Verification items for the finished model (mm, model axes). Face numbers are marked on the shaded views. A direction names the side the tool comes from. Round coordinates to 2 decimals unless told otherwise and drop trailing zeros. Order: outer loops, then holes, each group sorted by start corner. A loop starts at its lowest first (then second) coordinate and runs counter-clockwise, first axis right, second up.
```python
from build123d import *

# Parameters (mm, degrees)
SKETCH1_W             = 80
SKETCH1_H             = 40
SKETCH1_R             = 1.55
BOSS_EXTRUDE1_DEPTH   = 5
SKETCH1_W_2           = 40
SKETCH1_H_2           = 80
BOSS_EXTRUDE1_2_DEPTH = 5
BOSS_EXTRUDE1_3_DEPTH = 5
BOSS_EXTRUDE1_4_DEPTH = 5
SKETCH1_4_W           = 40
SKETCH1_4_H           = 40
BOSS_EXTRUDE2_DEPTH   = 310
CHAMFER1_SIZE         = 50
CHAMFER2_SIZE         = 50
BOSS_EXTRUDE3_START   = 180
SKETCH2_R             = 1.55
BOSS_EXTRUDE3_DEPTH   = 7.5
CHAMFER7_SIZE         = 10
SKETCH3_W             = 15
SKETCH3_H             = 15
BOSS_EXTRUDE4_DEPTH   = 20
SKETCH4_W             = 40
SKETCH4_H             = 22.28
BOSS_EXTRUDE5_DEPTH   = 5
CHAMFER8_SIZE         = 22
CHAMFER8_SIZE2        = 29.194986076


# Some blends are built 0.0001 mm under size
with BuildPart() as part:
    # Sketch1 → Boss-Extrude1 (new body)
    with BuildSketch(Plane(origin=(0, 0, 0), x_dir=(1, 0, 0), z_dir=(0, 1, 0))):
        with Locations((40, 20)):
            Rectangle(SKETCH1_W, SKETCH1_H)
        with Locations(Location((74, 6, 0), (0, 0, 270))):
            Circle(SKETCH1_R, mode=Mode.SUBTRACT)
        with Locations(Location((74, 34, 0), (0, 0, 270))):
            Circle(SKETCH1_R, mode=Mode.SUBTRACT)
    extrude(amount=BOSS_EXTRUDE1_DEPTH)



with BuildPart() as body_2:
    # Sketch1 → Boss-Extrude1 2 (new body)
    with BuildSketch(Plane(origin=(0, 0, 0), x_dir=(1, 0, 0), z_dir=(0, 1, 0))):
        with Locations((-20, 80)):
            Rectangle(SKETCH1_W_2, SKETCH1_H_2)
        with Locations(Location((-34, 114, 0), (0, 0, 270))):
            Circle(SKETCH1_R, mode=Mode.SUBTRACT)
        with Locations(Location((-6, 114, 0), (0, 0, 270))):
            Circle(SKETCH1_R, mode=Mode.SUBTRACT)
    extrude(amount=BOSS_EXTRUDE1_2_DEPTH)


with BuildPart() as body_3:
    # Sketch1 → Boss-Extrude1 3 (new body)
    with BuildSketch(Plane(origin=(0, 0, 0), x_dir=(1, 0, 0), z_dir=(0, 1, 0))):
        with Locations((-80, 20)):
            Rectangle(SKETCH1_W, SKETCH1_H)
        with Locations(Location((-114, 6, 0), (0, 0, 270))):
            Circle(SKETCH1_R, mode=Mode.SUBTRACT)
        with Locations(Location((-114, 34, 0), (0, 0, 270))):
            Circle(SKETCH1_R, mode=Mode.SUBTRACT)
    extrude(amount=BOSS_EXTRUDE1_3_DEPTH)


with BuildPart() as body_4:
    # Sketch1 → Boss-Extrude1 4 (new body)
    with BuildSketch(Plane(origin=(0, 0, 0), x_dir=(1, 0, 0), z_dir=(0, 1, 0))):
        with Locations((-20, -40)):
            Rectangle(SKETCH1_W_2, SKETCH1_H_2)
        with Locations(Location((-34, -74, 0), (0, 0, 270))):
            Circle(SKETCH1_R, mode=Mode.SUBTRACT)
        with Locations(Location((-6, -74, 0), (0, 0, 270))):
            Circle(SKETCH1_R, mode=Mode.SUBTRACT)
    extrude(amount=BOSS_EXTRUDE1_4_DEPTH)


with BuildPart() as part_1:
    add(part.part)

    add(body_2.part)  # Boss-Extrude2 merges body 2

    add(body_3.part)  # Boss-Extrude2 merges body 3

    add(body_4.part)  # Boss-Extrude2 merges body 4
    # Sketch1<4> → Boss-Extrude2 (add)
    with BuildSketch(Plane(origin=(0, 0, 0), x_dir=(1, 0, 0), z_dir=(0, 1, 0))):
        with Locations((-20, 20)):
            Rectangle(SKETCH1_4_W, SKETCH1_4_H)
    extrude(amount=BOSS_EXTRUDE2_DEPTH)

    # Chamfer1
    # the kernel refuses this chamfer: 50 mm, written as the material it adds along each edge
    with BuildSketch(Plane(origin=(0, 5, -40), x_dir=(1, 0, 0), z_dir=(0, 0, 1)), Plane(origin=(-40, 5, 0), x_dir=(-1, 0, 0), z_dir=(0, 0, -1))) as chamfer1_piece_1:
        Polygon((CHAMFER1_SIZE, 0), (0, CHAMFER1_SIZE), (0, 0), align=None)
    extrude(amount=40)

    # Chamfer2
    chamfer2_edges = [part_1.edges().sort_by_distance(p)[0] for p in [
        (-20, 5, -40),
        (-20, 5, 0),
    ]]
    chamfer(chamfer2_edges, length=CHAMFER2_SIZE - 0.0001)  # a hair under: the kernel refuses the full size

    # Sketch2 → Boss-Extrude3 (add)
    with BuildSketch(Plane(origin=(0, 0, 0), x_dir=(1, 0, 0), z_dir=(0, 1, 0)).offset(BOSS_EXTRUDE3_START)):
        Polygon((-64.25, 76.68), (-44.25, 76.68), (-44.25, 51.75), (-32.5, 40), (-7.5, 40), (4.25, 51.75), (4.25, 76.68), (24.25, 76.68), (24.25, 26.68), (-40, 26.68), (-64.25, 26.68), align=None)
        with Locations(Location((-54.25, 71.68, 0), (0, 0, 270))):
            Circle(SKETCH2_R, mode=Mode.SUBTRACT)
        with Locations(Location((14.25, 71.68, 0), (0, 0, 270))):
            Circle(SKETCH2_R, mode=Mode.SUBTRACT)
        with Locations(Location((-54.25, 31.68, 0), (0, 0, 270))):
            Circle(SKETCH2_R, mode=Mode.SUBTRACT)
        with Locations(Location((14.25, 31.68, 0), (0, 0, 270))):
            Circle(SKETCH2_R, mode=Mode.SUBTRACT)
    extrude(amount=BOSS_EXTRUDE3_DEPTH)

    # Chamfer7
    # the kernel refuses this chamfer: 10 mm, written as the material it adds along each edge
    with BuildSketch(Plane(origin=(-40, 187.5, -26.68), x_dir=(0, 1, 0), z_dir=(0, 0, -1))) as chamfer7_piece_1_section:
        Polygon((CHAMFER7_SIZE, 0), (0, -CHAMFER7_SIZE), (0, 0), align=None)
    chamfer7_piece_1 = extrude(amount=39.03682988, mode=Mode.PRIVATE)
    chamfer7_piece_1 = split(chamfer7_piece_1, bisect_by=Plane(origin=(-29.59, 187.5, -37.09), z_dir=(-0.7071067811865485, 0, 0.7071067811865467)), keep=Keep.TOP, mode=Mode.PRIVATE)
    chamfer7_piece_1 = split(chamfer7_piece_1, bisect_by=Plane(origin=(-40, 199.16, -38.34), z_dir=(0, -0.7071067811865476, 0.7071067811865476)), keep=Keep.TOP, mode=Mode.PRIVATE)
    add(chamfer7_piece_1)
    with BuildSketch(Plane(origin=(0, 187.5, -65.71682988), x_dir=(0, 1, 0), z_dir=(0, 0, 1))) as chamfer7_piece_2_section:
        Polygon((CHAMFER7_SIZE, 0), (0, -CHAMFER7_SIZE), (0, 0), align=None)
    chamfer7_piece_2 = extrude(amount=39.03682988, mode=Mode.PRIVATE)
    chamfer7_piece_2 = split(chamfer7_piece_2, bisect_by=Plane(origin=(9.10841494, 187.5, -56.60841494), z_dir=(0.7071067811865488, 0, 0.7071067811865462)), keep=Keep.TOP, mode=Mode.PRIVATE)
    chamfer7_piece_2 = split(chamfer7_piece_2, bisect_by=Plane(origin=(0, 179.64158506, -57.85841494), z_dir=(0, -0.7071067811865476, 0.7071067811865476)), keep=Keep.TOP, mode=Mode.PRIVATE)
    add(chamfer7_piece_2)
    with BuildSketch(Plane(origin=(-33.21682988, 187.5, -40), x_dir=(0, 1, 0), z_dir=(1, 0, 0))) as chamfer7_piece_3_section:
        Polygon((CHAMFER7_SIZE, 0), (0, -CHAMFER7_SIZE), (0, 0), align=None)
    chamfer7_piece_3 = extrude(amount=58.933659759, mode=Mode.PRIVATE)
    chamfer7_piece_3 = split(chamfer7_piece_3, bisect_by=Plane(origin=(-32.85841494, 187.5, -40.35841494), z_dir=(-0.7071067811865485, 0, 0.7071067811865467)), keep=Keep.TOP, mode=Mode.PRIVATE)
    add(chamfer7_piece_3)
    with BuildSketch(Plane(origin=(-33.21682988, 187.5, -40), x_dir=(0, 1, 0), z_dir=(1, 0, 0))) as chamfer7_piece_4_section:
        Polygon((CHAMFER7_SIZE, 0), (0, -CHAMFER7_SIZE), (0, 0), align=None)
    chamfer7_piece_4 = extrude(amount=58.933659759, mode=Mode.PRIVATE)
    chamfer7_piece_4 = split(chamfer7_piece_4, bisect_by=Plane(origin=(-20.35841494, 187.5, -27.14158506), z_dir=(0.7071067811865488, 0, 0.7071067811865462)), keep=Keep.TOP, mode=Mode.PRIVATE)
    chamfer7_piece_4 = split(chamfer7_piece_4, bisect_by=Plane(origin=(-11.60841494, 209.10841494, -40), z_dir=(-0.7071067811865476, -0.7071067811865476, 0)), keep=Keep.TOP, mode=Mode.PRIVATE)
    add(chamfer7_piece_4)
    with BuildSketch(Plane(origin=(-65.71682988, 187.5, -40), x_dir=(0, 1, 0), z_dir=(1, 0, 0))) as chamfer7_piece_5_section:
        Polygon((CHAMFER7_SIZE, 0), (0, -CHAMFER7_SIZE), (0, 0), align=None)
    chamfer7_piece_5 = extrude(amount=58.933659759, mode=Mode.PRIVATE)
    chamfer7_piece_5 = split(chamfer7_piece_5, bisect_by=Plane(origin=(-49.10841494, 187.5, -56.60841494), z_dir=(-0.7071067811865485, 0, 0.7071067811865467)), keep=Keep.TOP, mode=Mode.PRIVATE)
    chamfer7_piece_5 = split(chamfer7_piece_5, bisect_by=Plane(origin=(-57.85841494, 179.64158506, -40), z_dir=(0.7071067811865476, -0.7071067811865476, 0)), keep=Keep.TOP, mode=Mode.PRIVATE)
    add(chamfer7_piece_5)
    with BuildSketch(Plane(origin=(-65.71682988, 187.5, -40), x_dir=(0, 1, 0), z_dir=(1, 0, 0))) as chamfer7_piece_6_section:
        Polygon((CHAMFER7_SIZE, 0), (0, -CHAMFER7_SIZE), (0, 0), align=None)
    chamfer7_piece_6 = extrude(amount=58.933659759, mode=Mode.PRIVATE)
    chamfer7_piece_6 = split(chamfer7_piece_6, bisect_by=Plane(origin=(-36.60841494, 187.5, -10.89158506), z_dir=(0.7071067811865488, 0, 0.7071067811865462)), keep=Keep.TOP, mode=Mode.PRIVATE)
    add(chamfer7_piece_6)



with BuildPart() as body_2_2:
    # Sketch3 → Boss-Extrude4 (new body)
    with BuildSketch(Plane(origin=(0, 310, 0), x_dir=(1, 0, 0), z_dir=(0, 1, 0))):
        with Locations((-20, 54.78)):
            Rectangle(SKETCH3_W, SKETCH3_H)
    extrude(amount=BOSS_EXTRUDE4_DEPTH)


with BuildPart() as part_2:
    add(part_1.part)

    add(body_2_2.part)  # Boss-Extrude5 merges body 2 2
    # Sketch4 → Boss-Extrude5 (add)
    with BuildSketch(Plane(origin=(0, 310, 0), x_dir=(1, 0, 0), z_dir=(0, 1, 0))):
        with Locations((-20, 51.14)):
            Rectangle(SKETCH4_W, SKETCH4_H)
    extrude(amount=-BOSS_EXTRUDE5_DEPTH)

    # Chamfer8
    chamfer8_edges = [part_2.edges().sort_by_distance(p)[0] for p in [
        (-20, 305, -40),
    ]]
    chamfer8_side = [part_2.faces().sort_by_distance(p)[0] for p in [
        (-20, 305, -51.14),
    ]]
    chamfer(chamfer8_edges, length=CHAMFER8_SIZE, length2=CHAMFER8_SIZE2, reference=chamfer8_side[0])


solid = part_2.part
```
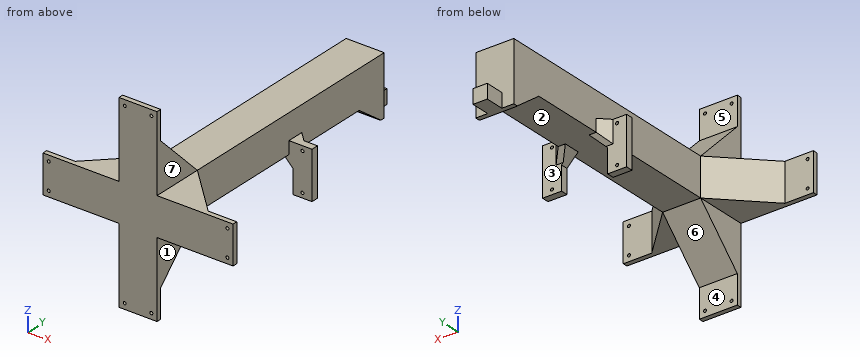
1) Sectioned sample at C-C on x = 42.5. Record the cut outline in (y, z), then the cut area to 3 significant figures.
2) Sectioned sample at A-A on x = 20.5. Record the cut outline in (y, z), then the cut area to 4 significant figures.
3) Go/stop test with flat-tipped pins: pin 1 Ø5 at (x, z) = (-34, 74) entering from +Y; pin 2 Ø4 at (x, y) = (-57, 185.5) entering from -Z; pin 3 Ø2 at (y, z) = (296.5, -34) entering from -X. Record where each tip stops, or that it passes through.
4) Draft check along Y on the marked faces 1, 2 and 3. Enter one of: released by +Y, released by -Y, zero draft, split by the parting line, or undercut.
5) Scan lines: probe 1 along X at (y, z) = (4, -114); probe 2 along X at (y, z) = (1, -34). Record each from-to range of solid material in increasing order.
6) Tool access check on the marked faces 4, 5, 6 and 7. Record the directions out of +Z, -Z, +X, -X, +Y, -Y that give a thin tool (end or side, any length) a straight path to the whole face; none if there is none.
7) Sectioned sample at D-D on y = 153. Record the cut outline in (x, z).
8) Sectioned sample at B-B on y = 48.5. Record the cut outline in (x, z), then the cut area to 3 significant figures.
Returned:
1. outline: (0, -40) - (12.5, -40) - (12.5, 0) - (0, 0) - close
1. area: 500 mm2
2. outline: (0, -40) - (34.5, -40) - (34.5, 0) - (0, 0) - close; (180, -76.68) - (187.5, -76.68) - (187.5, -26.68) - (180, -26.68) - close
2. area: 1,755 mm2
3. pin 1: stops at y = 5
3. pin 2: stops at z = -76.68
3. pin 3: stops at x = -40
4. face 1: zero draft
4. face 2: undercut
4. face 3: released by +Y
5. probe 1: x = -40 to -35.55, -32.45 to -7.55, -4.45 to 0
5. probe 2: x = -120 to -115.55, -112.45 to 72.45, 75.55 to 80
6. face 4: -Z, +X, -X, +Y
6. face 5: +Z, +X, -X, +Y
6. face 6: -Z, +X, -X
6. face 7: +Z, +X, +Y, -Y
7. outline: (-40, -40) - (0, -40) - (0, 0) - (-40, 0) - close
8. outline: (-46.5, -40) - (-40, -40) - (-40, -46.5) - (0, -46.5) - (0, -40) - (6.5, -40) - (6.5, 0) - (0, 0) - (0, 6.5) - (-40, 6.5) - (-40, 0) - (-46.5, 0) - close
8. area: 2,640 mm2
